Read the model definition and answer for the solid it produces. Units are mm, in the model's axes. Face numbers are marked on the shaded views. A direction names the side the tool comes from. Round coordinates to 2 decimals unless told otherwise and drop trailing zeros. Order: outer loops, then holes, each group sorted by start corner. A loop starts at its lowest first (then second) coordinate and runs counter-clockwise, first axis right, second up. Notation, with made-up numbers: (11, 17.25) -> (58, 17.25) arc R23 ccw to (58, 44.25) -> close; hole circle Ø7 at (-20.75, -26.75). An arc over 180 degrees is marked (long way). One line per item, written item: value. Start each with the question number.
1. Section B-B (x = 951) is taken. Give the vertices of the cut face in (y, z).
2. Section A-A (y = 477.5) is taken. Give the vertices of the cut face in (x, z), then the cut area to 3 significant figures.
3. Section C-C (z = 611) is taken. Give the vertices of the cut face in (x, y), then the cut area to 3 significant figures.
4. For the marked faces 1 and 2, determine the directions among +Z, -Z, +X, -X, +Y, -Y from which every point of the face is accessible in a straight line to the end or side of a thin tool.
5. A flat-ended cylindrical pin translates along its axis: pin 1 Ø2 at (x, y) = (614.5, 401) entering from +Z. Find the tip coordinate at first contact, or state that the pin passes through.
6. The mould has two halves that part along X. Classify the marked faces 3, 4 and 5: released by +X, released by -X, zero draft, split by the parting line, or undercut.
7. Consider line 1 (Z direction, x = 473, y = 562.5); line 2 (Y direction, x = 780.5, z = 443.5); line 3 (X direction, y = 301, z = 427). Determine where each line is inside the solid, lowest interval first.
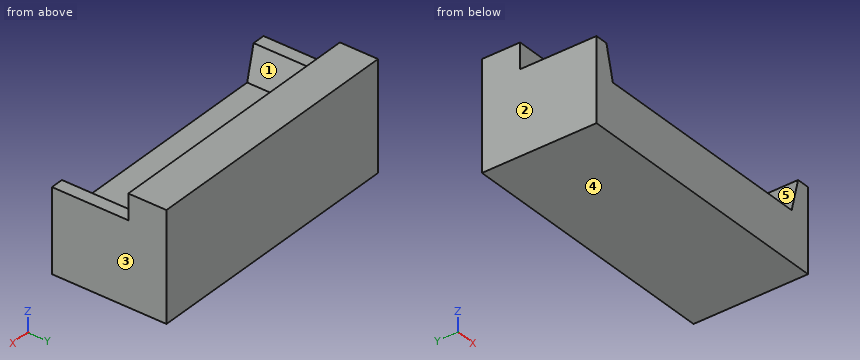
from build123d import *

# Parameters (mm, degrees)
SKETCH_W     = 2130
SKETCH_H     = 900
PAD_DEPTH    = 850
POCKET_DEPTH = 600


with BuildPart() as part:
    # Sketch → Pad (new body)
    with BuildSketch(Plane.XY):
        with Locations((1065, 450)):
            Rectangle(SKETCH_W, SKETCH_H)
    extrude(amount=PAD_DEPTH)

    # Sketch001 (on Face1 of Pad) → Pocket (cut)
    with BuildSketch(Plane.XZ):
        Polygon((0, 650), (100, 650), (164.921688, 390), (1965.078312, 390), (2030, 650), (2130, 650), (2130, 850), (0, 850), align=None)
    extrude(amount=-POCKET_DEPTH, mode=Mode.SUBTRACT)


solid = part.part
Answer:
1. outline: (0, 0) -> (900, 0) -> (900, 850) -> (600, 850) -> (600, 390) -> (0, 390) -> close
2. outline: (0, 0) -> (2130, 0) -> (2130, 650) -> (2030, 650) -> (1965.08, 390) -> (164.92, 390) -> (100, 650) -> (0, 650) -> close
2. area: 900,000 mm^2
3. outline: (0, 0) -> (109.74, 0) -> (109.74, 600) -> (2020.26, 600) -> (2020.26, 0) -> (2130, 0) -> (2130, 900) -> (0, 900) -> close
3. area: 771,000 mm^2
4. face 1: +Z, -Y
4. face 2: +Z, -Z, -X, +Y, -Y
5. pin 1: z = 390
6. face 3: released by +X
6. face 4: zero draft
6. face 5: undercut
7. line 1: 0 to 390
7. line 2: 600 to 900
7. line 3: 0 to 155.68, 1974.32 to 2130
